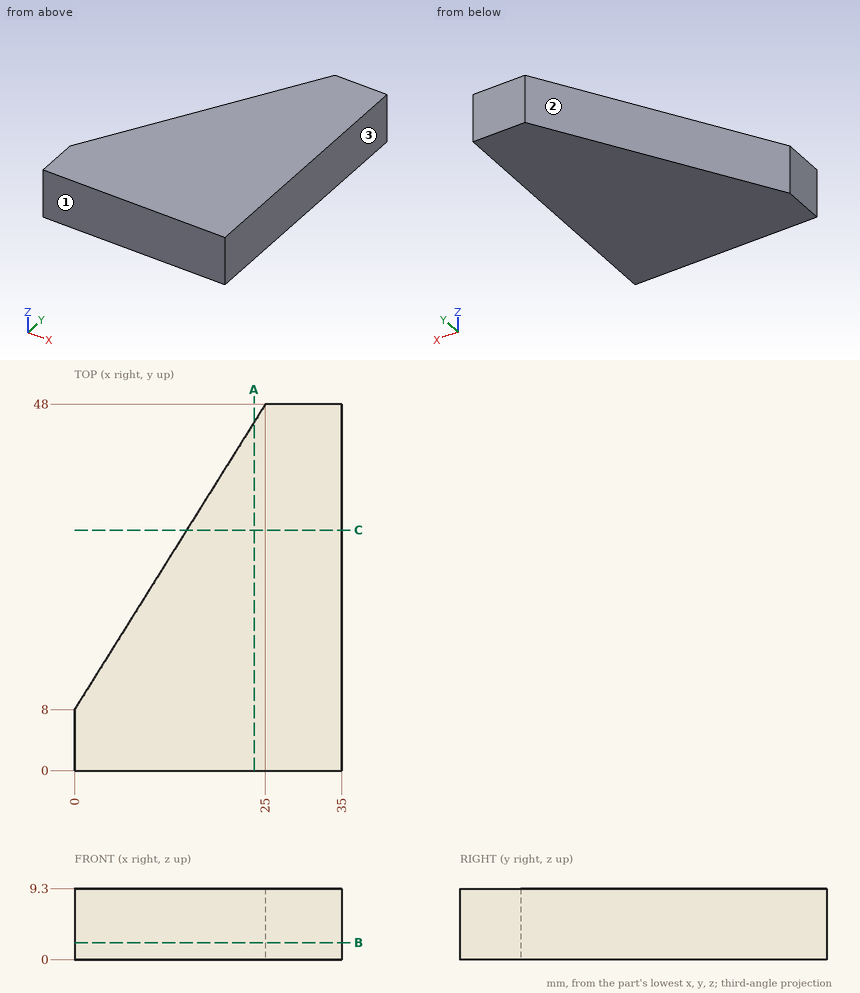
The drawing under review shows one solid part. Ordinate dimensions are in mm from its lowest x, y, z. Round coordinates to 2 decimals unless told otherwise and drop trailing zeros. Loops run counter-clockwise (first coordinate to the right, second up) from the corner with the lowest first, then second, coordinate; pieces in that order, holes last. Notation, with made-up numbers: (2, 86.5) - (15, 86.5) arc R20 ccw to (15, 94.5) - close; hole circle Ø10 at (67.5, 83.5). An arc over 180 degrees is marked (long way). Use a Markdown table: item, result. Add a question column.
Q1. Insertion check: pin 1 Ø5 at (x, z) = (10, 2) entering from +Y; pin 2 Ø1 at (y, z) = (34, 8.5) entering from -X; pin 3 Ø1.5 at (x, z) = (20.5, 7.5) entering from +Y. Each pin has a flat end and moves straight along its axis. Give the tip position at first contact, or say it passes through.
Q2. Add section B-B (z = 2.25). State the section outline as (x, y) points.
Q3. Add section C-C (y = 31.5). State the section outline as (x, z) points, plus the area to 3 significant figures.
Q4. For probe 1 along X at (y, z) = (21, 4) (3 decimals); probe 2 along X at (y, z) = (26.5, 8.5); probe 3 along Y at (x, z) = (8.5, 0.5), list the stretches that pass through material, from the lowest coordinate up.
Q5. Add section A-A (x = 23.5). State the section outline as (y, z) points, plus the area to 3 significant figures.
Q6. The part is to be moulded in two halves that separate along X. For the marked faces 1, 2 and 3, say which applies: pulls with the +X half, pulls with the -X half, needs draft (parallel to the pull), parting line crosses it, or undercut.
Worked answers:
| question | item | result |
|---|---|---|
| 1 | pin 1 | y = 28 |
| 1 | pin 2 | x = 15.94 |
| 1 | pin 3 | y = 42 |
| 2 | outline | (0, 0) - (35, 0) - (35, 48) - (25, 48) - (0, 8) - close |
| 3 | outline | (14.69, 0) - (35, 0) - (35, 9.3) - (14.69, 9.3) - close |
| 3 | area | 189 mm² |
| 4 | probe 1 | 8.125 to 35 |
| 4 | probe 2 | 11.56 to 35 |
| 4 | probe 3 | 0 to 21.6 |
| 5 | outline | (0, 0) - (45.6, 0) - (45.6, 9.3) - (0, 9.3) - close |
| 5 | area | 424 mm² |
| 6 | face 1 | needs draft |
| 6 | face 2 | pulls with the -X half |
| 6 | face 3 | pulls with the +X half |
